Can you work these out from the drawing? Everything is in mm from the part's minimum corner. Coordinates: 2 decimals unless noted, no trailing zeros. Loops run counter-clockwise (first coordinate to the right, second up) from the corner with the lowest first, then second, coordinate; pieces in that order, holes last.
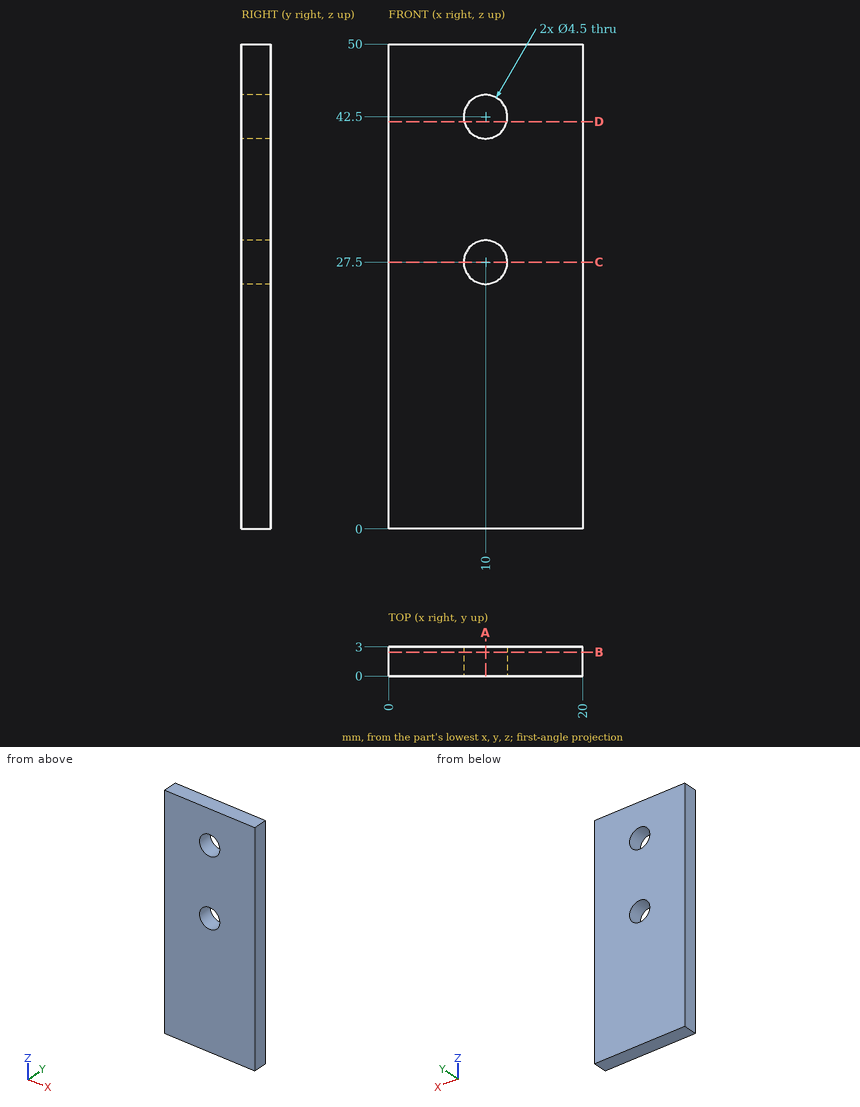
(1) Imagine slicing it at A-A, the plane x = 10. Write out the boundary of the cut face in (y, z), and give its area (3 significant figures).
Answers:
outline: (0, 0) - (3, 0) - (3, 25.25) - (0, 25.25) - close; (0, 29.75) - (3, 29.75) - (3, 40.25) - (0, 40.25) - close; (0, 44.75) - (3, 44.75) - (3, 50) - (0, 50) - close
area: 123 mm2
(2) I need wall thicknesses on probe 1 along Z at (x, y) = (10, 1.6); probe 2 along X at (y, z) = (0.7, 42.5); probe 3 along Z at (x, y) = (11, 2.25). Which ranges of each line are inside material? Lowest first, please.
Answers:
probe 1: z = 0 to 25.25, 29.75 to 40.25, 44.75 to 50
probe 2: x = 0 to 7.75, 12.25 to 20
probe 3: z = 0 to 25.48, 29.52 to 40.48, 44.52 to 50
(3) Imagine slicing it at B-B, the plane y = 2.45. Write out the boundary of the cut face in (x, z).
Answers:
outline: (0, 0) - (20, 0) - (20, 50) - (0, 50) - close; hole circle Ø4.5 at (10, 27.5); hole circle Ø4.5 at (10, 42.5)
(4) Imagine slicing it at C-C, the plane z = 27.5. Write out the boundary of the cut face in (x, y), and give its area (3 significant figures).
Answers:
outline: (0, 0) - (7.75, 0) - (7.75, 3) - (0, 3) - close; (12.25, 0) - (20, 0) - (20, 3) - (12.25, 3) - close
area: 46.5 mm2
(5) Imagine slicing it at D-D, the plane z = 42. Write out the boundary of the cut face in (x, y).
Answers:
outline: (0, 0) - (7.81, 0) - (7.81, 3) - (0, 3) - close; (12.19, 0) - (20, 0) - (20, 3) - (12.19, 3) - close
